Can you work these out from the drawing? Everything is in mm from the part's minimum corner. Round coordinates to 2 decimals unless told otherwise and drop trailing zeros. Loops run counter-clockwise (first coordinate to the right, second up) from the corner with the lowest first, then second, coordinate; pieces in that order, holes last. Notation, with made-up numbers: M 11.25,33 L 33.25,33 A11 ccw 33.25,51 Z; hole C -18.5,-38 d4. An arc over 180 degrees is marked long. Answer in a Markdown table with one row per item.
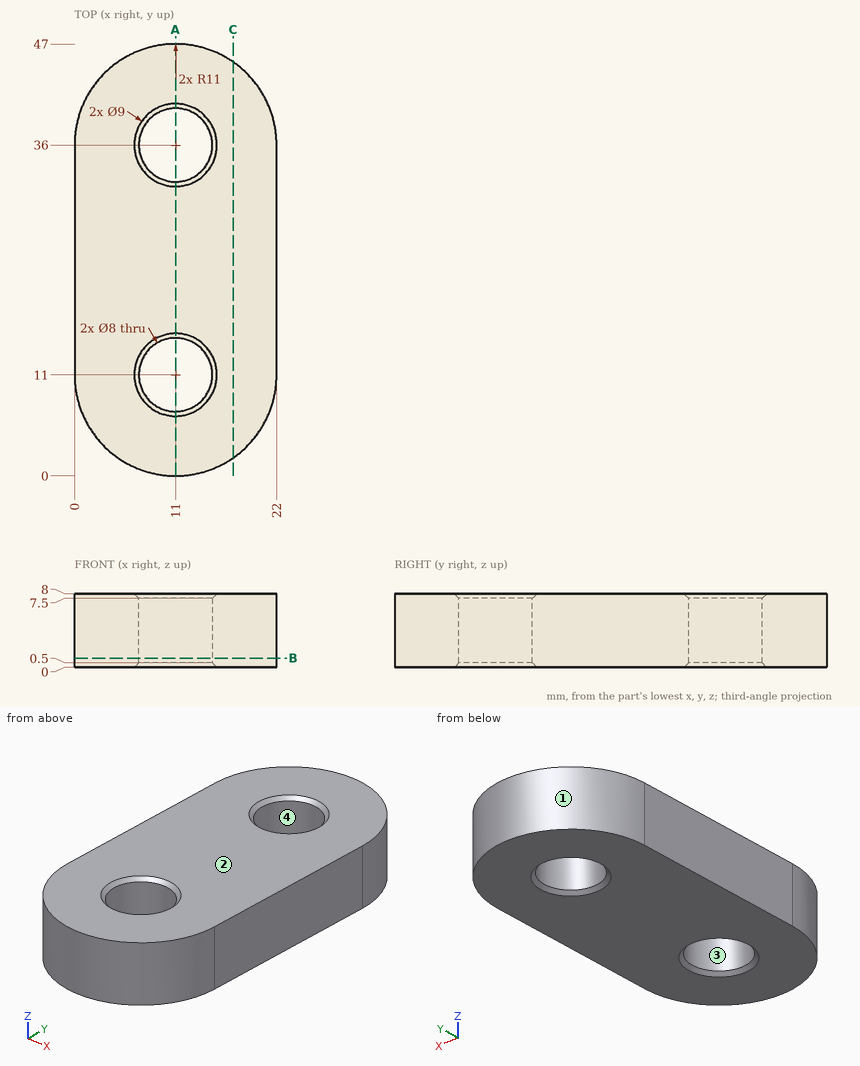
1) I need wall thicknesses on line 1 (Y direction, x = 11, z = 3); line 2 (Y direction, x = 9.5, z = 5.75); line 3 (X direction, y = 9.5, z = 4.5). Which ranges of each line are inside material? Lowest first, please.
Computed:
| item | result |
|---|---|
| line 1 | y = 0 to 7, 15 to 32, 40 to 47 |
| line 2 | y = 0.1 to 7.29, 14.71 to 32.29, 39.71 to 46.9 |
| line 3 | x = 0.1 to 7.29, 14.71 to 21.9 |
2) Will this pin go through, and if not, where does the flat tip stop? P1, Ø1.5, axis at x = 5.5, z = 2.5, coming from the -Y side.
Computed:
| item | result |
|---|---|
| P1 | stops at y = 1.08 |
3) I want a section at B-B, the plane z = 1. Please give me the cut outline in (x, y), plus the area to 3 significant figures.
Computed:
| item | result |
|---|---|
| outline | M 0,11 A11 ccw 22,11 L 22,36 A11 ccw 0,36 Z; hole C 11,11 d8; hole C 11,36 d8 |
| area | 830 mm² |
4) I want a section at C-C, the plane x = 17.25. Please give me the cut outline in (y, z), plus the area to 3 significant figures.
Computed:
| item | result |
|---|---|
| outline | M 1.95,0 L 45.05,0 L 45.05,8 L 1.95,8 Z |
| area | 345 mm² |
5) If we mould it in two halves opening along Y, with no side actions, what happens to the marked faces 1, 2, 3 and 4? For each: released by +Y, released by -Y, zero draft, split by the parting line, or undercut.
Computed:
| item | result |
|---|---|
| face 1 | released by +Y |
| face 2 | zero draft |
| face 3 | undercut |
| face 4 | undercut |
6) I want a section at A-A, the plane x = 11. Please give me the cut outline in (y, z), plus the area to 3 significant figures.
Computed:
| item | result |
|---|---|
| outline | M 0,0 L 6.5,0 L 7,0.5 L 7,7.5 L 6.5,8 L 0,8 Z; M 15,0.5 L 15.5,0 L 31.5,0 L 32,0.5 L 32,7.5 L 31.5,8 L 15.5,8 L 15,7.5 Z; M 40,0.5 L 40.5,0 L 47,0 L 47,8 L 40.5,8 L 40,7.5 Z |
| area | 247 mm² |
